For this review, take the finished solid that the model builds, in its own axes (mm). Face numbers are marked on the shaded views. A direction names the side the tool comes from. Coordinates: 2 decimals unless noted, no trailing zeros.
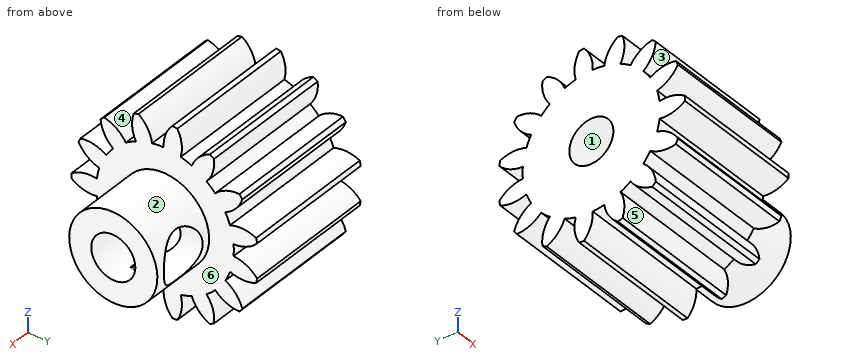
```python
from build123d import *

# Parameters (mm, degrees)
SPUR_START             = -93.736960043
SPUR_GEAR_AI_OUTLINE_R = 1.5875
SPUR_GEAR_AI_DEPTH     = 9.525
SKETCH1_R              = 3.175
SKETCH1_R_2            = 1.5875
BOSS_EXTRUDE1_DEPTH    = 4.7625
SKETCH2_R              = 1.7859375
CUT_EXTRUDE1_DEPTH     = 3.175


# Read off the part's stored shape, not the designer's step: spur gear_ai
with BuildPart() as part:
    # spur gear_ai outline → spur gear_ai (new body)
    with BuildSketch(Plane.YZ.offset(SPUR_START)):
        with BuildLine():
            ThreePointArc((26.294144563, 31.128016902), (26.400392113, 31.270279151), (26.502859253, 31.415288028))
            ThreePointArc((26.502859253, 31.415288028), (26.037760207, 32.257629699), (25.277278274, 32.847141228))
            ThreePointArc((25.277278274, 32.847141228), (25.463945724, 33.222717571), (25.618148436, 33.612748146))
            ThreePointArc((25.618148436, 33.612748146), (26.565102615, 33.44206014), (27.502296476, 33.660060783))
            ThreePointArc((27.502296476, 33.660060783), (27.541495173, 33.833238586), (27.576123139, 34.007387928))
            ThreePointArc((27.576123139, 34.007387928), (26.808622795, 34.58773251), (25.874112039, 34.816962221))
            ThreePointArc((25.874112039, 34.816962221), (25.891880579, 35.235992775), (25.874112039, 35.655023329))
            ThreePointArc((25.874112039, 35.655023329), (26.808622795, 35.88425304), (27.576123139, 36.464597623))
            ThreePointArc((27.576123139, 36.464597623), (27.541495173, 36.638746964), (27.502296476, 36.811924767))
            ThreePointArc((27.502296476, 36.811924767), (26.565102615, 37.029925411), (25.618148436, 36.859237404))
            ThreePointArc((25.618148436, 36.859237404), (25.463945724, 37.249267979), (25.277278274, 37.624844322))
            ThreePointArc((25.277278274, 37.624844322), (26.037760207, 38.214355851), (26.502859253, 39.056697522))
            ThreePointArc((26.502859253, 39.056697522), (26.400392113, 39.201706399), (26.294144563, 39.343968648))
            ThreePointArc((26.294144563, 39.343968648), (25.349306519, 39.161931061), (24.553645896, 38.620838844))
            ThreePointArc((24.553645896, 38.620838844), (24.254134982, 38.914429611), (23.930845121, 39.181611181))
            ThreePointArc((23.930845121, 39.181611181), (24.385803996, 40.029472629), (24.468081893, 40.988162861))
            ThreePointArc((24.468081893, 40.988162861), (24.315493079, 41.078957921), (24.160567843, 41.165706181))
            ThreePointArc((24.160567843, 41.165706181), (23.371456696, 40.615106316), (22.864666581, 39.797169648))
            ThreePointArc((22.864666581, 39.797169648), (22.471635623, 39.943556096), (22.067623104, 40.056144773))
            ThreePointArc((22.067623104, 40.056144773), (22.138392398, 41.015753193), (21.823622551, 41.925025735))
            ThreePointArc((21.823622551, 41.925025735), (21.647296055, 41.945907688), (21.470481113, 41.962142396))
            ThreePointArc((21.470481113, 41.962142396), (20.97354135, 41.138183972), (20.843250357, 40.184831534))
            ThreePointArc((20.843250357, 40.184831534), (20.424657978, 40.158702116), (20.009780236, 40.097230294))
            ThreePointArc((20.009780236, 40.097230294), (19.684123296, 41.002660673), (19.02673227, 41.705294043))
            ThreePointArc((19.02673227, 41.705294043), (18.857156545, 41.652652209), (18.689024808, 41.595566237))
            ThreePointArc((18.689024808, 41.595566237), (18.570181828, 40.64071915), (18.838918453, 39.716794239))
            ThreePointArc((18.838918453, 39.716794239), (18.467143079, 39.522666969), (18.113136244, 39.297763686))
            ThreePointArc((18.113136244, 39.297763686), (17.447362113, 39.992458885), (16.56101879, 40.366961389))
            ThreePointArc((16.56101879, 40.366961389), (16.427515019, 40.24989802), (16.297137991, 40.129362051))
            ThreePointArc((16.297137991, 40.129362051), (16.576940826, 39.208728037), (17.198238065, 38.473985665))
            ThreePointArc((17.198238065, 38.473985665), (16.937563035, 38.145426912), (16.705638106, 37.795979987))
            ThreePointArc((16.705638106, 37.795979987), (15.81486518, 38.159820895), (14.852826371, 38.141437649))
            ThreePointArc((14.852826371, 38.141437649), (14.778478569, 37.980194064), (14.708399623, 37.817049862))
            ThreePointArc((14.708399623, 37.817049862), (15.33846782, 37.089814907), (16.204897737, 36.671298704))
            ThreePointArc((16.204897737, 36.671298704), (16.100396131, 36.26511926), (16.030655035, 35.851551242))
            ThreePointArc((16.030655035, 35.851551242), (15.068906044, 35.821626462), (14.197517, 35.413536095))
            ThreePointArc((14.197517, 35.413536095), (14.195180579, 35.235992775), (14.197517, 35.058449455))
            ThreePointArc((14.197517, 35.058449455), (15.068906044, 34.650359089), (16.030655035, 34.620434308))
            ThreePointArc((16.030655035, 34.620434308), (16.100396131, 34.20686629), (16.204897737, 33.800686847))
            ThreePointArc((16.204897737, 33.800686847), (15.33846782, 33.382170643), (14.708399623, 32.654935688))
            ThreePointArc((14.708399623, 32.654935688), (14.778478569, 32.491791486), (14.852826371, 32.330547901))
            ThreePointArc((14.852826371, 32.330547901), (15.81486518, 32.312164655), (16.705638106, 32.676005564))
            ThreePointArc((16.705638106, 32.676005564), (16.937563035, 32.326558639), (17.198238065, 31.997999885))
            ThreePointArc((17.198238065, 31.997999885), (16.576940826, 31.263257513), (16.297137991, 30.3426235))
            ThreePointArc((16.297137991, 30.3426235), (16.427515019, 30.222087531), (16.56101879, 30.105024161))
            ThreePointArc((16.56101879, 30.105024161), (17.447362114, 30.479526665), (18.113136244, 31.174221865))
            ThreePointArc((18.113136244, 31.174221865), (18.467143079, 30.949318581), (18.838918453, 30.755191311))
            ThreePointArc((18.838918453, 30.755191311), (18.570181828, 29.831266401), (18.689024808, 28.876419314))
            ThreePointArc((18.689024808, 28.876419314), (18.857156545, 28.819333342), (19.02673227, 28.766691508))
            ThreePointArc((19.02673227, 28.766691508), (19.684123296, 29.469324877), (20.009780236, 30.374755256))
            ThreePointArc((20.009780236, 30.374755256), (20.424657978, 30.313283434), (20.843250357, 30.287154017))
            ThreePointArc((20.843250357, 30.287154017), (20.97354135, 29.333801579), (21.470481113, 28.509843154))
            ThreePointArc((21.470481113, 28.509843154), (21.647296055, 28.526077862), (21.823622551, 28.546959815))
            ThreePointArc((21.823622551, 28.546959815), (22.138392398, 29.456232358), (22.067623104, 30.415840778))
            ThreePointArc((22.067623104, 30.415840778), (22.471635623, 30.528429454), (22.864666581, 30.674815902))
            ThreePointArc((22.864666581, 30.674815902), (23.371456696, 29.856879235), (24.160567843, 29.30627937))
            ThreePointArc((24.160567843, 29.30627937), (24.315493079, 29.393027629), (24.468081893, 29.483822689))
            ThreePointArc((24.468081893, 29.483822689), (24.385803996, 30.442512921), (23.930845121, 31.290374369))
            ThreePointArc((23.930845121, 31.290374369), (24.254134982, 31.557555939), (24.553645896, 31.851146706))
            ThreePointArc((24.553645896, 31.851146706), (25.349306519, 31.310054489), (26.294144563, 31.128016902))
        make_face()
        with Locations((20.942055579, 35.235992775)):
            Circle(SPUR_GEAR_AI_OUTLINE_R, mode=Mode.SUBTRACT)
    extrude(amount=SPUR_GEAR_AI_DEPTH)

    # Sketch1 → Boss-Extrude1 (add)
    with BuildSketch(Plane(origin=(-84.211960043, 0, 0), x_dir=(0, 0, -1), z_dir=(1, 0, 0))):
        with Locations(Location((-35.235992775, 20.942055579, 0), (0, 0, 180))):
            Circle(SKETCH1_R)
        with Locations((-35.235992775, 20.942055579)):
            Circle(SKETCH1_R_2, mode=Mode.SUBTRACT)
    extrude(amount=BOSS_EXTRUDE1_DEPTH)

    # Sketch2 → Cut-Extrude1 (cut)
    with BuildSketch(Plane(origin=(0, 24.117055579, 0), x_dir=(1, 0, 0), z_dir=(0, 1, 0))):
        with Locations(Location((-81.830710043, -35.235992775, 0), (0, 0, 270))):
            Circle(SKETCH2_R)
    extrude(amount=-CUT_EXTRUDE1_DEPTH, mode=Mode.SUBTRACT)


solid = part.part
```
Q1. Machinability: for the marked faces 4, 5 and 6, which of the approach directions +Z, -Z, +X, -X, +Y, -Y give a long, thin tool a straight path to every point of the face, cutting with its end or side? Answer none if there is none.
Q2. Wall thickness on probe 1 along X at (y, z) = (16.5, 30.75); probe 2 along Y at (x, z) = (-89.5, 35.5); probe 3 along Y at (x, z) = (-90.5, 36.5): over which ranges is each line inside the solid? List them lowest first.
Q3. The part is to be moulded in two halves that separate along Y. For the marked faces 1, 2 and 3, say which applies: +Y half, -Y half, draft (parallel to the pull), parting line (faces both ways), or undercut.
Q4. For pin 1 Ø6 at (x, y) = (-90.5, 19.5) entering from -Z; pin 2 Ø3 at (x, z) = (-83, 37) entering from -Y; pin 3 Ø4 at (x, y) = (-87, 26) entering from -Z; pin 4 Ø4 at (x, z) = (-82, 30) entering from -Y, all flat-tipped, find the tip position at first contact; note any pin that passes through.
Model answer:
1. face 4: +Z, +X, -X
1. face 5: +X, -X
1. face 6: +X
2. probe 1: x = -93.74 to -84.21
2. probe 2: y = 14.32 to 19.38, 22.51 to 25.88
2. probe 3: y = 16.16 to 19.98, 21.9 to 27.57
3. face 1: undercut
3. face 2: parting line
3. face 3: -Y half
4. pin 1: stops at z = 28.51
4. pin 2: stops at y = 14.71
4. pin 3: stops at z = 29.31
4. pin 4: passes through
